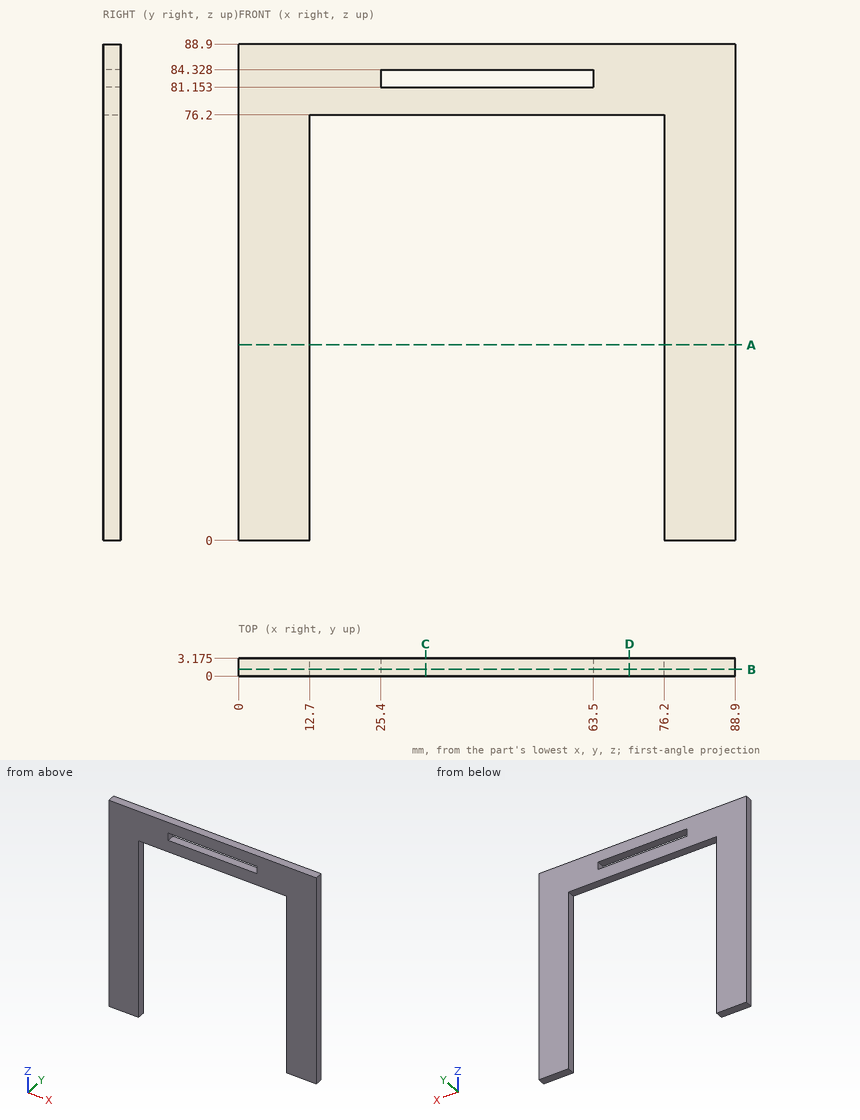
For this review, use the dimensioned drawing (mm, ordinates from the lowest corner) and the shaded views. Coordinates: 2 decimals unless noted, no trailing zeros. Order: outer loops, then holes, each group sorted by start corner. A loop starts at its lowest first (then second) coordinate and runs counter-clockwise, first axis right, second up. Notation, with made-up numbers: M 7,40.25 L 22,40.25 A22 cw 22,72.25 Z; hole C 31,43 d11. An arc over 180 degrees is marked long. Answer as a JSON object with one key per item and string values. Group by question number.
1) Add section B-B, the plane y = 1.2. Write out the cut boundary in (x, z), then the cut area to 3 significant figures.
2) For pin 1 (1 mm diameter, centred on x = 41.5, y = 1, fed in from -Z); pin 2 (1 mm diameter, centred on x = 77, z = 18.5, fed in from -Y), all flat-tipped, find the tip position at first contact; note any pin that passes through.
3) Add section A-A, the plane z = 35. Write out the cut boundary in (x, y) (3 decimals), then the cut area to 3 significant figures.
4) Add section C-C, the plane x = 33.5. Write out the cut boundary in (y, z) (3 decimals), then the cut area to 3 significant figures.
5) Add section D-D, the plane x = 70. Write out the cut boundary in (y, z) (3 decimals), then the cut area to 3 significant figures.
6) Wall thickness on L1, parallel to Z at x = 33, y = 0.85; L2, parallel to X at y = 1.4, z = 37; L3, parallel to Z at x = 20, y = 1.9: over which ranges is each line inside the solid? List them lowest first.
Computed values:
{
 "1": {"outline": "M 0,0 L 12.7,0 L 12.7,76.2 L 76.2,76.2 L 76.2,0 L 88.9,0 L 88.9,88.9 L 0,88.9 Z; hole M 25.4,81.15 L 63.5,81.15 L 63.5,84.33 L 25.4,84.33 Z", "area": "2,940 mm^2"},
 "2": {"pin 1": "stops at z = 76.2", "pin 2": "stops at y = 0"},
 "3": {"outline": "M 0,0 L 12.7,0 L 12.7,3.175 L 0,3.175 Z; M 76.2,0 L 88.9,0 L 88.9,3.175 L 76.2,3.175 Z", "area": "80.6 mm^2"},
 "4": {"outline": "M 0,76.2 L 3.175,76.2 L 3.175,81.153 L 0,81.153 Z; M 0,84.328 L 3.175,84.328 L 3.175,88.9 L 0,88.9 Z", "area": "30.2 mm^2"},
 "5": {"outline": "M 0,76.2 L 3.175,76.2 L 3.175,88.9 L 0,88.9 Z", "area": "40.3 mm^2"},
 "6": {"L1": "z = 76.2 to 81.15, 84.33 to 88.9", "L2": "x = 0 to 12.7, 76.2 to 88.9", "L3": "z = 76.2 to 88.9"}
}
